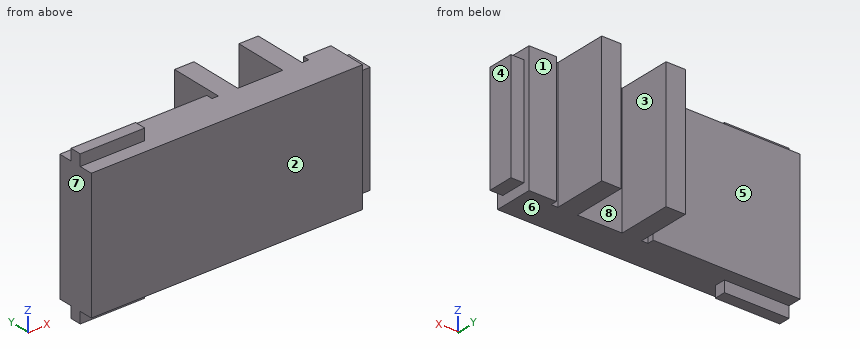
```python
from build123d import *

# Parameters (mm, degrees)
BOSS_EXTRUDE1_DEPTH = 20
SKETCH6_W           = 17
SKETCH6_H           = 4
BOSS_EXTRUDE3_DEPTH = 2
SKETCH7_W           = 3
SKETCH7_H           = 20
BOSS_EXTRUDE4_DEPTH = 8.35
SKETCH8_W           = 1.75
SKETCH8_H           = 1.75
BOSS_EXTRUDE5_DEPTH = 10


with BuildPart() as part:
    # Sketch2 → Boss-Extrude1 (new body)
    with BuildSketch(Plane.XY):
        Polygon((-7.5, 1), (-30.26, 1), (-30.26, -5), (11.75, -5), (11.75, 1), (7.5, 1), (7.5, 0), (-7.5, 0), align=None)
    extrude(amount=BOSS_EXTRUDE1_DEPTH)

    # Sketch6 → Boss-Extrude3 (add)
    with BuildSketch(Plane(origin=(11.75, 0, 0), x_dir=(0, 0, -1), z_dir=(1, 0, 0))):
        with Locations((-10, -2)):
            Rectangle(SKETCH6_W, SKETCH6_H)
    extrude(amount=BOSS_EXTRUDE3_DEPTH)

    # Sketch7 → Boss-Extrude4 (add)
    with BuildSketch(Plane(origin=(0, 0, 0), x_dir=(1, 0, 0), z_dir=(0, 1, 0))):
        with Locations((-5, -10)):
            Rectangle(SKETCH7_W, SKETCH7_H)
        with Locations((4.965868183, -10)):
            Rectangle(SKETCH7_W, SKETCH7_H)
    extrude(amount=BOSS_EXTRUDE4_DEPTH)

    # Sketch8 → Boss-Extrude5 (add)
    with BuildSketch(Plane.ZY.offset(30.26)):
        with Locations((-0.875, -2)):
            Rectangle(SKETCH8_W, SKETCH8_H)
        with Locations((20.875, -2)):
            Rectangle(SKETCH8_W, SKETCH8_H)
    extrude(amount=-BOSS_EXTRUDE5_DEPTH)


solid = part.part
```
Geometry: final body of the model. Coordinates: model frame, mm. Face numbers are marked on the shaded views. A direction names the side the tool comes from. Coordinates: 2 decimals unless noted, no trailing zeros. Loops run counter-clockwise (first coordinate to the right, second up) from the corner with the lowest first, then second, coordinate; pieces in that order, holes last. Notation, with made-up numbers: M 69,-13.5 L 128,-13.5 A28 ccw 128,5.5 Z; hole C 61.5,29.25 d10. An arc over 180 degrees is marked long. Put each result on its own line as item: value.
(1) Access query for the marked faces 1, 2, 3, 4 and 5. Directions: +Z, -Z, +X, -X, +Y, -Y. A direction counts if a zero-diameter tool reaches every point of the face in a straight line with its end or side. Return the directions, or none.
Answer sheet:
face 1: +Z, -Z, +X, +Y
face 2: +Z, -Z, +X, -X, -Y
face 3: +Z, -Z, +Y
face 4: +Z, -Z, +X, +Y, -Y
face 5: +Z, -Z, -X, +Y
(2) Cut plane A-A on z = 8.25. Return the cut outline in (x, y).
Answer sheet:
outline: M -30.26,-5 L 11.75,-5 L 11.75,-4 L 13.75,-4 L 13.75,0 L 11.75,0 L 11.75,1 L 7.5,1 L 7.5,0 L 6.47,0 L 6.47,8.35 L 3.47,8.35 L 3.47,0 L -3.5,0 L -3.5,8.35 L -6.5,8.35 L -6.5,0 L -7.5,0 L -7.5,1 L -30.26,1 Z
(3) Cut plane C-C on x = -27.5. Return the cut outline in (y, z) (3 decimals).
Answer sheet:
outline: M -5,0 L -2.875,0 L -2.875,-1.75 L -1.125,-1.75 L -1.125,0 L 1,0 L 1,20 L -1.125,20 L -1.125,21.75 L -2.875,21.75 L -2.875,20 L -5,20 Z
(4) Material intervals for probe 1 along X at (y, z) = (2.25, 7); probe 2 along Z at (x, y) = (11.5, -1.5); probe 3 along Y at (x, z) = (-27.5, -0.5) (3 decimals), sorted ascending.
Answer sheet:
probe 1: x = -6.5 to -3.5, 3.47 to 6.47
probe 2: z = 0 to 20
probe 3: y = -2.875 to -1.125
(5) Draft query along X for the marked faces 6, 7 and 8. Return one class per face: pulls with the +X half, pulls with the -X half, needs draft (parallel to the pull), parting line crosses it, or undercut.
Answer sheet:
face 6: needs draft
face 7: pulls with the -X half
face 8: undercut
(6) Cut plane B-B on y = 3.75. Return the cut outline in (x, z).
Answer sheet:
outline: M -6.5,0 L -3.5,0 L -3.5,20 L -6.5,20 Z; M 3.47,0 L 6.47,0 L 6.47,20 L 3.47,20 Z
(7) Cut plane D-D on y = -2. Return the cut outline in (x, z), then the cut area to 3 significant figures.
Answer sheet:
outline: M -30.26,-1.75 L -20.26,-1.75 L -20.26,0 L 11.75,0 L 11.75,1.5 L 13.75,1.5 L 13.75,18.5 L 11.75,18.5 L 11.75,20 L -20.26,20 L -20.26,21.75 L -30.26,21.75 Z
area: 909 mm^2
(8) First-contact query: pin 1 (0.9 mm diameter, centred on y = -2, z = 21, fed in from +X); pin 2 (2 mm diameter, centred on x = 13, y = -2, fed in from +Z); pin 3 (0.5 mm diameter, centred on x = -23.5, z = 21, fed in from +Y) (3 decimals); pin 4 (1.6 mm diameter, centred on x = 12.5, z = 6, fed in from -Y). Flat tips, straight axial feed; report the tip coordinate or a pass-through.
Answer sheet:
pin 1: stops at x = -20.26
pin 2: stops at z = 18.5
pin 3: stops at y = -1.125
pin 4: stops at y = -5
